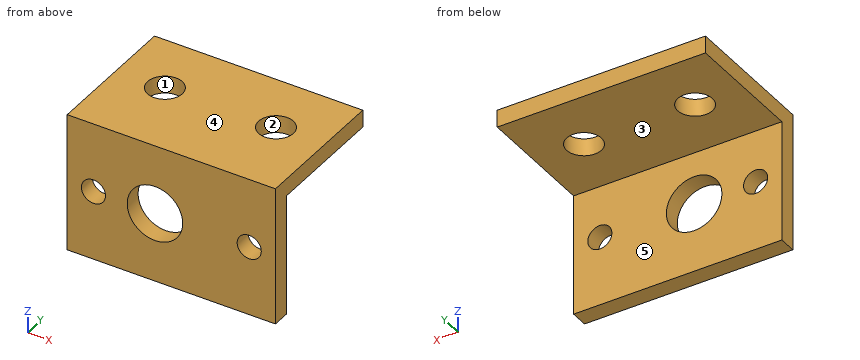
Autodesk Inventor part; units mm, degrees
ref_plane "YZ Plane" through (0, 0, 0) normal (1, 0, 0) x (0, 1, 0)
ref_plane "XZ Plane" through (0, 0, 0) normal (0, 1, 0) x (-1, 0, 0)
ref_plane "XY Plane" through (0, 0, 0) normal (0, 0, 1) x (1, 0, 0)
sketch "Sketch1" plane through (0, 0, 0) normal (1, 0, 0) x (0, 1, 0)
  line L0 (0, 0) -> (25.4, 0)
  line L1 (25.4, 0) -> (25.4, -25.4)
  line L2 (25.4, -25.4) -> (0, -25.4)
  line L3 (0, -25.4) -> (0, 0)
  line L4 (0, -25.4) -> (3.175, -25.4)
  line L5 (25.4, 0) -> (25.4, -3.175)
  line L6 (25.4, -3.175) -> (3.175, -3.175)
  line L7 (3.175, -3.175) -> (3.175, -25.4)
  dimension "d0" = 25.4
  dimension "d1" = 25.4
  dimension "d2" = 3.175
  dimension "d3" = 3.175
extrude "Extrusion1" add sketch "Sketch1" along normal blind 38.1 contours L0 L1 L6 L7 L2 L3
sketch "Sketch2" plane through (0, 3.175, -3.175) normal (0, 1, 0) x (1, 0, 0)
  line L0 (0, -3.175) -> (0, 22.225) construction
  line L1 (0, 22.225) -> (0, -3.175) construction
  line L2 (0, 9.525) -> (38.1, 9.525) construction
  line L3 (38.1, -3.175) -> (38.1, 22.225) construction
  circle A0 centre (4.8006, 9.525) radius 2.206
  circle A1 centre (33.2994, 9.525) radius 2.206
  line L4 (33.2994, 9.525) -> (19.05, 9.525) construction
  line L5 (19.05, 9.525) -> (4.8006, 9.525) construction
  line L6 (4.8006, 9.525) -> (16.0528, 9.525) construction
  circle A2 centre (16.0528, 9.525) radius 5.08
  dimension "d6" = 25.4
  dimension "d7" = 14.2494
  dimension "d8" = 14.2494
  dimension "d11" = 4.412
  dimension "d12" = 4.412
  dimension "d13" = 11.2522
  dimension "d15" = 10.16
extrude "Extrusion2" cut sketch "Sketch2" against normal blind 38.1
sketch "Sketch3" plane through (0, 3.175, -3.175) normal (0, 0, -1) x (-1, 0, 0)
  line L0 (0, 22.225) -> (0, -3.175) construction
  line L1 (0, 22.225) -> (0, 0) construction
  line L2 (0, 11.1125) -> (-38.1, 11.1125) construction
  line L3 (-38.1, 0) -> (-38.1, 22.225) construction
  circle A0 centre (-29.21, 11.1125) radius 3.175
  circle A1 centre (-8.89, 11.1125) radius 3.175
  line L4 (-19.05, 11.1125) -> (-19.05, 13.4043) construction
  dimension "d16" = 22.225
  dimension "d17" = 10.16
  dimension "d18" = 10.16
  dimension "d19" = 6.35
  dimension "d20" = 6.35
extrude "Extrusion3" cut sketch "Sketch3" against normal blind 38.1
equation "\"d0\" = d1"
equation "\"d8\" = d7"
equation "\"d12\" = d11"
equation "\"d18\" = d17"
equation "\"d20\" = d19"
properties part number "bumper bracket"
Can you work these out from the model? Positions are in its coordinate system, mm. Face numbers are marked on the shaded views. A direction names the side the tool comes from. Give positions to 0.01 mm unless a question says otherwise; leave off trailing zeros. Loops run counter-clockwise (first coordinate to the right, second up) from the corner with the lowest first, then second, coordinate; pieces in that order, holes last. Notation, with made-up numbers: M -18.75,-34 L 40.25,-34 A12 ccw 40.25,-21 Z; hole C 29,30.25 d11. An arc over 180 degrees is marked long. One line per item, written item: value. Start each with the question number.
1) On a 3-axis mill with a long thin cutter (end or side, diameter ignored), from which of +Z, -Z, +X, -X, +Y, -Y can I reach the whole of each face in a straight line? I mean the marked faces 4 and 5. Say none if no direction works.
2) If we section it at C-C, the plane y = 15: Write out the boundary of the cut face in (x, z) (3 decimals).
3) Thinking about a two-plate mould opening in X: for the marked faces 1, 2 and 3, which applies, +X half, -X half, draft (parallel to the pull), parting line (faces both ways), or undercut?
4) If I drill on line 1 (X direction, y = 1.95, z = -12.7); line 2 (X direction, y = 16.75, z = -1.75); line 3 (Y direction, x = 6, z = -5) (3 decimals), over which ranges is the centre line in solid material (lowest first)? Write a range as [from, to].
5) I'm going to push flat-ended pins straight in: pin 1 (6 mm diameter, centred on x = 16.05, z = -12.7, fed in from -Y); pin 2 (1.5 mm diameter, centred on x = 6.5, y = 7, fed in from -Z) (3 decimals); pin 3 (6 mm diameter, centred on x = 17, z = -15, fed in from +Y) (3 decimals). Where does each tip first touch, or does it pass through?
6) If we section it at A-A, the plane z = -12.7: Write out the boundary of the cut face in (x, y) (3 decimals).
7) If we section it at D-D, the plane x = 19.5: Write out the boundary of the cut face in (y, z) (3 decimals).
8) If we section it at B-B, the plane x = 8.89: Write out the boundary of the cut face in (y, z) (1 decimal), and give its area (3 significant figures).
Completed:
1. face 4: +Z, +X, -X, +Y, -Y
1. face 5: -Z, +X, -X, +Y
2. outline: M 0,-3.175 L 5.796,-3.175 L 5.796,0 L 0,0 Z; M 11.984,-3.175 L 26.116,-3.175 L 26.116,0 L 11.984,0 Z; M 32.304,-3.175 L 38.1,-3.175 L 38.1,0 L 32.304,0 Z
3. face 1: undercut
3. face 2: undercut
3. face 3: draft
4. line 1: x = [0, 2.59], [7.01, 10.97], [21.13, 31.09], [35.51, 38.1]
4. line 2: x = [0, 6.89], [10.89, 27.21], [31.21, 38.1]
4. line 3: y = [0, 3.175]
5. pin 1: passes through
5. pin 2: stops at z = -3.175
5. pin 3: stops at y = 3.175
6. outline: M 0,0 L 2.595,0 L 2.595,3.175 L 0,3.175 Z; M 7.007,0 L 10.973,0 L 10.973,3.175 L 7.007,3.175 Z; M 21.133,0 L 31.093,0 L 31.093,3.175 L 21.133,3.175 Z; M 35.505,0 L 38.1,0 L 38.1,3.175 L 35.505,3.175 Z
7. outline: M 0,-25.4 L 3.175,-25.4 L 3.175,-16.431 L 0,-16.431 Z; M 0,-8.969 L 3.175,-8.969 L 3.175,-3.175 L 25.4,-3.175 L 25.4,0 L 0,0 Z
8. outline: M 0,-25.4 L 3.2,-25.4 L 3.2,-3.2 L 11.1,-3.2 L 11.1,0 L 0,0 Z; M 17.5,-3.2 L 25.4,-3.2 L 25.4,0 L 17.5,0 Z
8. area: 131 mm^2
